For this review, take the finished solid that the model builds, in its own axes (mm). A direction names the side the tool comes from. Coordinates: 2 decimals unless noted, no trailing zeros. Loops run counter-clockwise (first coordinate to the right, second up) from the corner with the lowest first, then second, coordinate; pieces in that order, holes last. Notation, with made-up numbers: (72, 78.25) -> (114, 78.25) arc R10 ccw to (114, 86.25) -> close; hole circle Ø4 at (5, 29). An arc over 180 degrees is marked (long way). Use a Markdown table: item, result.
from build123d import *

# Parameters (mm, degrees)
SKETCH1_W           = 71.12
SKETCH1_H           = 109.22
BOSS_EXTRUDE1_DEPTH = 6.35
BOSS_EXTRUDE3_DEPTH = 6.35
FILLET1_R           = 6.35
SKETCH3_W           = 19.05
SKETCH3_H           = 6.35
CUT_EXTRUDE1_DEPTH  = 6.35


with BuildPart() as part:
    # Sketch1 → Boss-Extrude1 (new body)
    with BuildSketch(Plane(origin=(0, 0, 0), x_dir=(1, 0, 0), z_dir=(0, 1, 0))):
        with BuildLine():
            Line((-40.159459459, 57.460725462), (36.040540541, 57.460725462))
            ThreePointArc((36.040540541, 57.460725462), (39.632642989, 55.972827911), (41.120540541, 52.380725462))
            Line((41.120540541, 52.380725462), (41.120540541, -61.919274538))
            ThreePointArc((41.120540541, -61.919274538), (39.632642989, -65.511376986), (36.040540541, -66.999274538))
            Line((36.040540541, -66.999274538), (-40.159459459, -66.999274538))
            ThreePointArc((-40.159459459, -66.999274538), (-43.751561908, -65.511376986), (-45.239459459, -61.919274538))
            Line((-45.239459459, -61.919274538), (-45.239459459, 52.380725462))
            ThreePointArc((-45.239459459, 52.380725462), (-43.751561908, 55.972827911), (-40.159459459, 57.460725462))
        make_face()
        with Locations((-2.059459459, -4.769274538)):
            Rectangle(SKETCH1_W, SKETCH1_H, mode=Mode.SUBTRACT)
    extrude(amount=-BOSS_EXTRUDE1_DEPTH)

    # Sketch1<4> → Boss-Extrude3 (add)
    with BuildSketch(Plane(origin=(0, 0, 0), x_dir=(1, 0, 0), z_dir=(0, 1, 0))):
        with BuildLine():
            Line((-40.159459459, 65.080725462), (36.040540541, 65.080725462))
            ThreePointArc((36.040540541, 65.080725462), (45.020796662, 61.360981583), (48.740540541, 52.380725462))
            Line((48.740540541, 52.380725462), (48.740540541, -61.919274538))
            ThreePointArc((48.740540541, -61.919274538), (45.020796662, -70.899530659), (36.040540541, -74.619274538))
            Line((36.040540541, -74.619274538), (-40.159459459, -74.619274538))
            ThreePointArc((-40.159459459, -74.619274538), (-49.139715581, -70.899530659), (-52.859459459, -61.919274538))
            Line((-52.859459459, -61.919274538), (-52.859459459, 52.380725462))
            ThreePointArc((-52.859459459, 52.380725462), (-49.139715581, 61.360981583), (-40.159459459, 65.080725462))
        make_face()
    extrude(amount=BOSS_EXTRUDE3_DEPTH)

    # Fillet1
    fillet1_edges = [part.edges().sort_by_distance(p)[0] for p in [
        (-49.139715581, 6.35, -61.360981583),
        (-2.059459459, 6.35, -65.080725462),
        (45.020796662, 6.35, -61.360981583),
        (48.740540541, 6.35, 4.769274538),
        (45.020796662, 6.35, 70.899530659),
        (-2.059459459, 6.35, 74.619274538),
        (-49.139715581, 6.35, 70.899530659),
        (-52.859459459, 6.35, 4.769274538),
    ]]
    fillet(fillet1_edges, radius=FILLET1_R - 0.0001)  # a hair under: the kernel refuses the full size

    # Sketch3 → Cut-Extrude1 (cut)
    with BuildSketch(Plane.XY.offset(74.619274538)):
        with Locations((-2.059459459, 0)):
            Rectangle(SKETCH3_W, SKETCH3_H)
    extrude(amount=-CUT_EXTRUDE1_DEPTH, mode=Mode.SUBTRACT)


solid = part.part
(1) Mouldability with a two-part tool opening along Z and no side actions: class faces 1 (the face through (-3, -3, -49.841)), 2 (the face through (33.501, -3, 6)), 3 (the face through (7.466, 2, 71)), 4 (the face through (-2, -3, 66.999)) as pulls with the +Z half, pulls with the -Z half, needs draft (parallel to the pull), parting line crosses it, or undercut.
Found:
| item | result |
|---|---|
| face 1 | undercut |
| face 2 | undercut |
| face 3 | needs draft |
| face 4 | pulls with the +Z half |
(2) For line 1 along X through (y, z) = (-4, 14.5); line 2 along Z through (x, y) = (28, -4.5); line 3 along Y through (x, z) = (-20, -6.5), list the stretches that pass through material, from the lowest coordinate up.
Found:
| item | result |
|---|---|
| line 1 | x = -45.24 to -37.62, 33.5 to 41.12 |
| line 2 | z = -57.46 to -49.84, 59.38 to 67 |
| line 3 | y = 0 to 6.35 |
(3) For faces 5 (the face through (39.672, -3.131, 65.472)), 6 (the face through (-2, 3.175, 71)), 7 (the face through (41.121, -3, 4)), list the 3-axis set-ups (+Z, -Z, +X, -X, +Y, -Y) from which the entire face can be reached by the end or side of a thin tool; tool diameter is ignored.
Found:
| item | result |
|---|---|
| face 5 | +Z, +X, -Y |
| face 6 | +Z, -Y |
| face 7 | +Z, -Z, +X, -Y |
(4) Take a section at A-A on y = -4. Write out the cut boundary in (x, z).
Found:
| item | result |
|---|---|
| outline | (-45.24, -52.38) arc R5.08 ccw to (-40.16, -57.46) -> (36.04, -57.46) arc R5.08 ccw to (41.12, -52.38) -> (41.12, 61.92) arc R5.08 ccw to (36.04, 67) -> (-40.16, 67) arc R5.08 ccw to (-45.24, 61.92) -> close; hole (-37.62, -49.84) -> (33.5, -49.84) -> (33.5, 59.38) -> (-37.62, 59.38) -> close |
(5) For pin 1 Ø7 at (y, z) = (-4.5, 0) entering from +X; pin 2 Ø5 at (x, y) = (-15.5, 5) entering from +Z; pin 3 Ø1.6 at (y, z) = (1.5, 72.5) entering from -X, all flat-tipped, find the tip position at first contact; note any pin that passes through.
Found:
| item | result |
|---|---|
| pin 1 | stops at x = 41.12 |
| pin 2 | stops at z = 74.11 |
| pin 3 | stops at x = -48.02 |
